```python
from build123d import *

# Parameters (mm, degrees)
ESBO_O1_R                = 4
ESBO_O1_R_2              = 3
RESSALTO_EXTRUS_O1_DEPTH = 10
ESBO_O2_W                = 8
ESBO_O2_H                = 4
RESSALTO_EXTRUS_O2_DEPTH = 10


with BuildPart() as part:
    # Esboço1 → Ressalto-extrusão1 (new body)
    with BuildSketch(Plane.XY):
        Circle(ESBO_O1_R)
        Circle(ESBO_O1_R_2, mode=Mode.SUBTRACT)
    extrude(amount=RESSALTO_EXTRUS_O1_DEPTH)

    # Esboço2 → Ressalto-extrusão2 (add)
    with BuildSketch(Plane(origin=(0, 0, 0), x_dir=(-1, 0, 0), z_dir=(0, 0, -1))):
        with Locations((0, -2)):
            Rectangle(ESBO_O2_W, ESBO_O2_H)
    extrude(amount=RESSALTO_EXTRUS_O2_DEPTH)


solid = part.part
```
Input: part model. Units: mm. Frame: model coordinates. A direction names the side the tool comes from. Round coordinates to 2 decimals unless told otherwise and drop trailing zeros. Loops run counter-clockwise (first coordinate to the right, second up) from the corner with the lowest first, then second, coordinate; pieces in that order, holes last. Notation, with made-up numbers: (26.25, 10.25) -> (58.25, 10.25) arc R17 ccw to (58.25, 24.25) -> close; hole circle Ø11 at (82, -33). An arc over 180 degrees is marked (long way). One line per item, written item: value.
(1) Set-up query: faces 4 (the face through (0, 0, -5)), 5 (the face through (3, -3, 0)), 6 (the face through (-3, -3, 0)), 7 (the face through (-0.867, -3.905, 4.93)). Return all of +Z, -Z, +X, -X, +Y, -Y with unobstructed straight access to the full face (end or side cutting, diameter ignored); none if empty.
Geometry check:
face 4: -Z, +X, -X, +Y
face 5: +Z, +X, -Y
face 6: +Z, -X, -Y
face 7: +Z
(2) Section A-A (x = -1.5). Return the cut outline in (y, z), plus the area to 3 significant figures.
Geometry check:
outline: (-4, -10) -> (0, -10) -> (0, 0) -> (-2.6, 0) -> (-2.6, 10) -> (-3.71, 10) -> (-3.71, 0) -> (-4, 0) -> close; (2.6, 0) -> (3.71, 0) -> (3.71, 10) -> (2.6, 10) -> close
area: 62.2 mm2
(3) Section C-C (y = -2.75). Return the cut outline in (x, z).
Geometry check:
outline: (-4, -10) -> (4, -10) -> (4, 0) -> (2.9, 0) -> (2.9, 10) -> (1.2, 10) -> (1.2, 0) -> (-1.2, 0) -> (-1.2, 10) -> (-2.9, 10) -> (-2.9, 0) -> (-4, 0) -> close
(4) Section D-D (z = 2). Return the cut outline in (x, y), plus the area to 3 significant figures.
Geometry check:
outline: circle Ø8 at (0, 0); hole circle Ø6 at (0, 0)
area: 22.0 mm2
(5) Pin query (flat end, axial travel): pin 1 (1 mm diameter, centred on x = 0.5, y = -1.5, fed in from +Z); pin 2 (4 mm diameter, centred on x = 1.5, z = -7, fed in from +Y). Return the tip coordinate at first contact, or that it passes through.
Geometry check:
pin 1: z = 0
pin 2: y = 0
(6) Mould query, pull axis Y, two halves, no side actions, for faces 1 (the face through (0, -4, -5)), 2 (the face through (0, -1, 0)), 3 (the face through (4, -2, -5)). Classes: pulls with the +Y half, pulls with the -Y half, needs draft (parallel to the pull), parting line crosses it, or undercut.
Geometry check:
face 1: pulls with the -Y half
face 2: undercut
face 3: needs draft
(7) Section B-B (y = 1.75). Return the cut outline in (x, z), plus the area to 3 significant figures.
Geometry check:
outline: (-3.6, 0) -> (-2.44, 0) -> (-2.44, 10) -> (-3.6, 10) -> close; (2.44, 0) -> (3.6, 0) -> (3.6, 10) -> (2.44, 10) -> close
area: 23.2 mm2
(8) Material intervals for line 1 (Y direction, x = 0, z = 5.25); line 2 (Y direction, x = -1.25, z = -5.5), sorted ascending. Write a range as [from, to].
Geometry check:
line 1: [-4, -3], [3, 4]
line 2: [-4, 0]
